For this review, use the dimensioned drawing (mm, ordinates from the lowest corner) and the shaded views. A direction names the side the tool comes from. Coordinates: 2 decimals unless noted, no trailing zeros. Loops run counter-clockwise (first coordinate to the right, second up) from the corner with the lowest first, then second, coordinate; pieces in that order, holes last. Notation, with made-up numbers: (82, -29.5) -> (106, -29.5) arc R28 cw to (106, 6.5) -> close; hole circle Ø8 at (-21, -37.5). An arc over 180 degrees is marked (long way). Use one line per item in the form item = value. Start each with the question number.
1. Consider section C-C (y = 2.75). State the section outline as (x, z) points.
2. Machinability: for the marked faces 1 and 2, which of the approach directions +Z, -Z, +X, -X, +Y, -Y give a long, thin tool a straight path to every point of the face, cutting with its end or side? Answer none if there is none.
3. Consider section D-D (y = 9.5). State the section outline as (x, z) points, then the cut area to 3 significant figures.
4. Consider section B-B (x = 7). State the section outline as (y, z) points.
5. The part is to be moulded in two halves that separate along Y. For the marked faces 3, 4 and 5, say which applies: released by +Y, released by -Y, zero draft, split by the parting line, or undercut.
6. Wall thickness on line 1 (Y direction, x = 3.5, z = 3.1); line 2 (Y direction, x = 8, z = 2.5); line 3 (Z direction, x = 5, y = 13.5): over which ranges is each line inside the solid? List them lowest first. Write a range as from..to.
7. Consider section A-A (z = 4). State the section outline as (x, y) points.
8. For pin 1 (5.5 mm diameter, centred on x = 7, y = 15, fed in from +Z); pin 2 (3 mm diameter, centred on x = 12, y = 6.5, fed in from +Z); pin 3 (1.5 mm diameter, centred on x = 2, z = 5, fed in from +Y), all flat-tipped, find the tip position at first contact; note any pin that passes through.
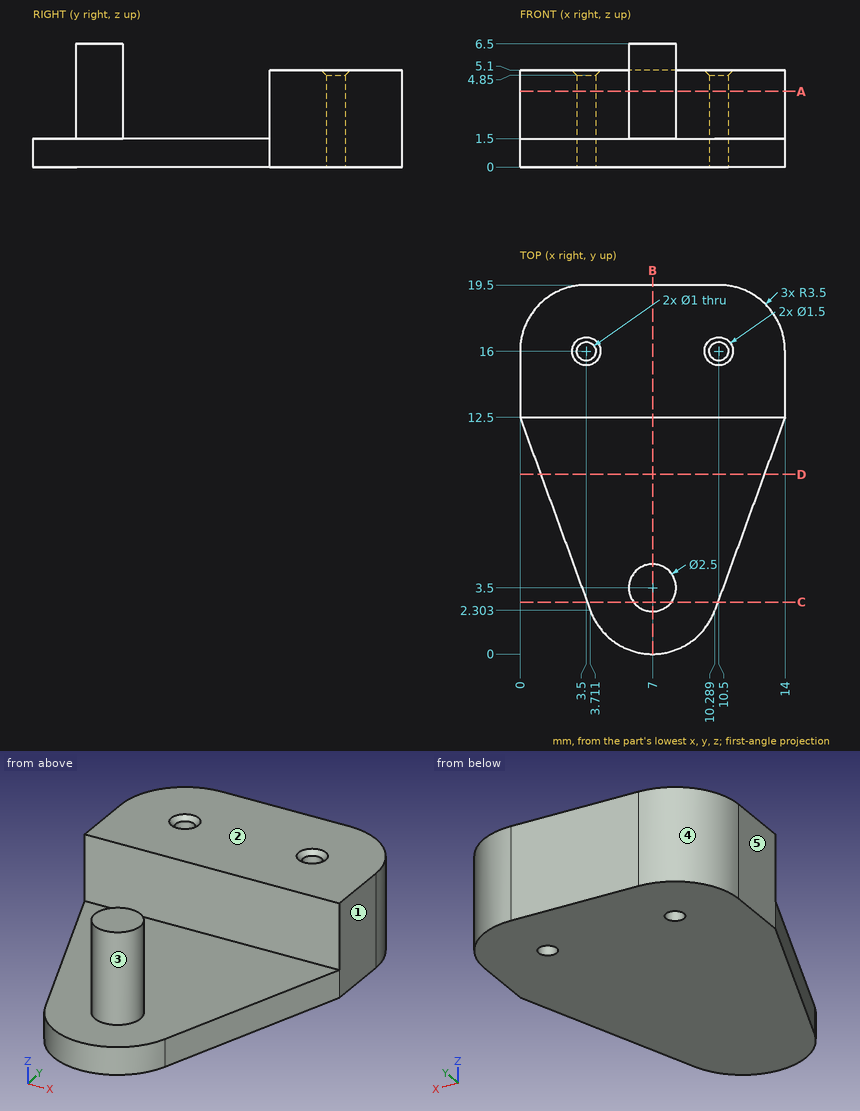
Geometry check:
q1.outline = (3.55, 0) -> (10.45, 0) -> (10.45, 1.5) -> (8, 1.5) -> (8, 6.5) -> (6, 6.5) -> (6, 1.5) -> (3.55, 1.5) -> close
q2.face_1 = +Z, -Z, +X, +Y, -Y
q2.face_2 = +Z, +X, -X, +Y
q3.outline = (1.09, 0) -> (12.91, 0) -> (12.91, 1.5) -> (1.09, 1.5) -> close
q3.area = 17.7 mm²
q4.outline = (0, 0) -> (19.5, 0) -> (19.5, 5.1) -> (12.5, 5.1) -> (12.5, 1.5) -> (4.75, 1.5) -> (4.75, 6.5) -> (2.25, 6.5) -> (2.25, 1.5) -> (0, 1.5) -> close
q5.face_3 = undercut
q5.face_4 = released by +Y
q5.face_5 = zero draft
q6.line_1 = 12.5..15.5, 16.5..19.5
q6.line_2 = 2.75..4.25, 12.5..19.5
q6.line_3 = 0..5.1
q7.outline = (0, 12.5) -> (14, 12.5) -> (14, 16) arc R3.5 ccw to (10.5, 19.5) -> (3.5, 19.5) arc R3.5 ccw to (0, 16) -> close; circle Ø2.5 at (7, 3.5); hole circle Ø1 at (3.5, 16); hole circle Ø1 at (10.5, 16)
q8.pin_1 = 5.1
q8.pin_2 = 1.5
q8.pin_3 = 19.42
